Could you check a few things on this drawing? It's one solid part, dimensions in mm from its lowest x, y, z. Give positions to 0.01 mm unless a question says otherwise; leave off trailing zeros. Order: outer loops, then holes, each group sorted by start corner. A loop starts at its lowest first (then second) coordinate and runs counter-clockwise, first axis right, second up. Notation, with made-up numbers: (60.25, -18.75) -> (89.25, -18.75) arc R13 cw to (89.25, -7.75) -> close; hole circle Ø4 at (-26.75, -19.5). An arc over 180 degrees is marked (long way). Answer as a JSON object with one key per item and string values.
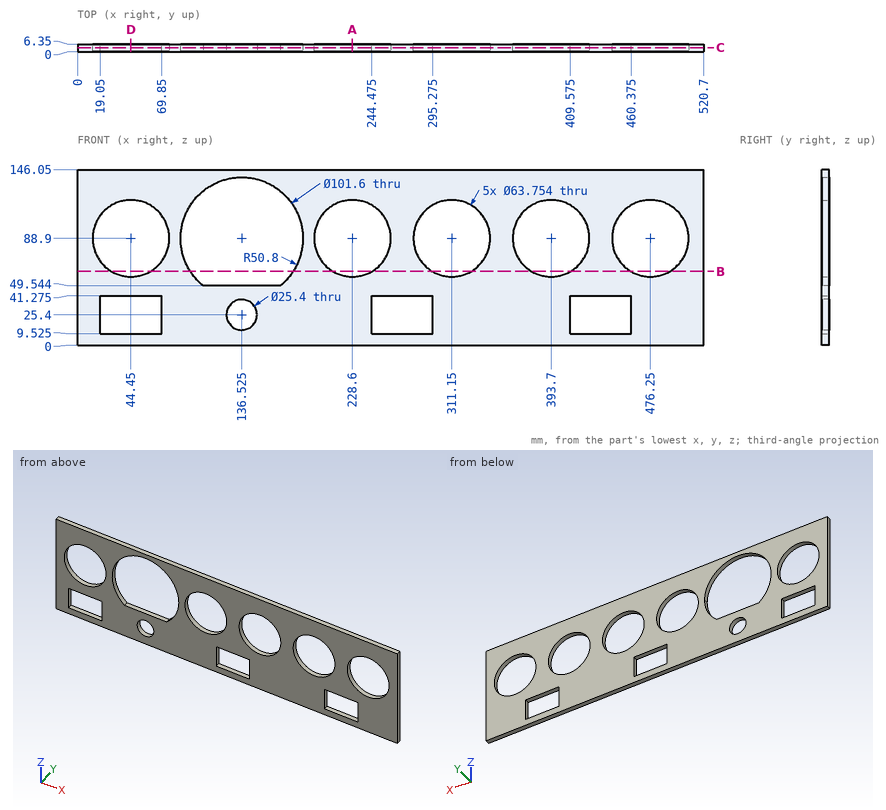
1. Please list where these lines run through material, in increasing order: L1, parallel to X at y = 5.5, z = 39.5 (3 decimals); L2, parallel to Z at x = 311.15, y = 3.75; L3, parallel to Z at x = 44.45, y = 2.25 (3 decimals).
Worked answers:
{"L1": "0 to 19.05, 69.85 to 244.475, 295.275 to 409.575, 460.375 to 520.7", "L2": "0 to 57.02, 120.78 to 146.05", "L3": "0 to 9.525, 41.275 to 57.023, 120.777 to 146.05"}
2. If we section it at B-B on z = 61.5: Please give me the cut outline in (x, y), then the cut area to 3 significant figures.
Worked answers:
{"outline": "(0, 0) -> (28.16, 0) -> (28.16, 6.35) -> (0, 6.35) -> close; (60.74, 0) -> (93.75, 0) -> (93.75, 6.35) -> (60.74, 6.35) -> close; (179.3, 0) -> (212.31, 0) -> (212.31, 6.35) -> (179.3, 6.35) -> close; (244.89, 0) -> (294.86, 0) -> (294.86, 6.35) -> (244.89, 6.35) -> close; (327.44, 0) -> (377.41, 0) -> (377.41, 6.35) -> (327.44, 6.35) -> close; (409.99, 0) -> (459.96, 0) -> (459.96, 6.35) -> (409.99, 6.35) -> close; (492.54, 0) -> (520.7, 0) -> (520.7, 6.35) -> (492.54, 6.35) -> close", "area": "1,730 mm²"}
3. If we section it at C-C on y = 3.25: Count the separate pieces of the cut face and the enclosed holes in it, then the cut area to 3 significant figures.
Worked answers:
{"separate pieces": "1", "enclosed holes": "10", "area": "47,100 mm²"}
4. If we section it at A-A on x = 228.6: Please give me the cut outline in (y, z).
Worked answers:
{"outline": "(0, 0) -> (6.35, 0) -> (6.35, 57.02) -> (0, 57.02) -> close; (0, 120.78) -> (6.35, 120.78) -> (6.35, 146.05) -> (0, 146.05) -> close"}
5. If we section it at D-D on x = 44.45: Please give me the cut outline in (y, z) (3 decimals).
Worked answers:
{"outline": "(0, 0) -> (6.35, 0) -> (6.35, 9.525) -> (0, 9.525) -> close; (0, 41.275) -> (6.35, 41.275) -> (6.35, 57.023) -> (0, 57.023) -> close; (0, 120.777) -> (6.35, 120.777) -> (6.35, 146.05) -> (0, 146.05) -> close"}
